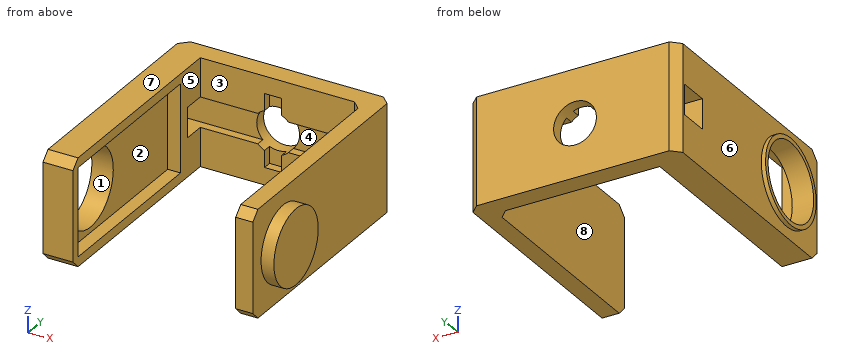
Autodesk Inventor part; units mm, degrees
ref_plane "YZ Plane" through (0, 0, 0) normal (1, 0, 0) x (0, 1, 0)
ref_plane "XZ Plane" through (0, 0, 0) normal (0, 1, 0) x (-1, 0, 0)
ref_plane "XY Plane" through (0, 0, 0) normal (0, 0, 1) x (1, 0, 0)
sketch "Boceto1" plane through (0, 0, 0) normal (0, 0, 1) x (1, 0, 0)
  line L0 (-12, 0) -> (-16, 0)
  line L1 (-16, 0) -> (-16, 55)
  line L2 (-16, 55) -> (-12, 55)
  line L3 (-12, 55) -> (-12, 0)
  line L4 (-12, 55) -> (-62, 55)
  line L5 (-62, 55) -> (-62, 50.3)
  line L6 (-62, 50.3) -> (-12, 50.3)
  line L7 (-12, 50.3) -> (-12, 55)
  line L8 (-62, 55) -> (-58, 55)
  line L9 (-58, 55) -> (-58, 0)
  line L10 (-58, 0) -> (-62, 0)
  line L11 (-62, 0) -> (-62, 55)
  dimension "d4" = 4
  dimension "d5" = 55
  dimension "d6" = 50
  dimension "d7" = 4.7
  dimension "d8" = 4
  dimension "d9" = 55
extrude "Extrusión1" add sketch "Boceto1" along normal blind 25
sketch "Boceto2" plane through (-58, 0, 0) normal (1, 0, 0) x (0, 0, -1)
  line L0 (-25, 0) -> (-25, 50.3)
  circle A0 centre (-12.5, 12) radius 9
  line L1 (0, 0) -> (-25, 0)
  dimension "d12" = 12.5
  dimension "d13" = 18
  dimension "d21" = 12
extrude "Extrusión2" cut sketch "Boceto2" against normal blind 15
sketch "Boceto3" plane through (-12, 0, 0) normal (1, 0, 0) x (0, 0, -1)
  line L0 (0, 0) -> (0, 55)
  line L1 (0, 0) -> (-25, 0)
  circle A0 centre (-12.5, 12) radius 8.75
  dimension "d16" = 17.5
  dimension "d17" = 12
  dimension "d18" = 12.5
extrude "Extrusión3" add sketch "Boceto3" along normal blind 3
sketch "Boceto4" plane through (-58, 0, 0) normal (1, 0, 0) x (0, 0, -1)
  circle A0 centre (-12.5, 12) radius 9
  line L0 (0, 50.3) -> (-25, 50.3)
  line L1 (-25, 0) -> (-25, 50.3)
  line L2 (0, 0) -> (-25, 0)
  line L3 (0, 0) -> (0, 50.3)
extrude "Extrusión4" add sketch "Boceto4" along normal blind 4
sketch "Boceto7" plane through (-62, 55, 0) normal (0, 1, 0) x (1, 0, 0)
  line L0 (50, 0) -> (0, 0)
  circle A0 centre (25, -12.5) radius 5
  line L1 (6.5, -9) -> (43.5, -9)
  line L2 (43.5, -9) -> (43.5, -16)
  line L3 (43.5, -16) -> (6.5, -16)
  line L4 (6.5, -16) -> (6.5, -9)
  line L5 (23, -4) -> (27, -4)
  line L6 (27, -4) -> (27, -21)
  line L7 (27, -21) -> (23, -21)
  line L8 (23, -21) -> (23, -4)
  line L9 (50, 0) -> (0, 0)
  point P0 (58, 0)
  point P1 (6.5, -12.5)
  point P2 (25, -9)
  point P3 (23, -12.5)
  point P4 (25, -4)
  point P5 (25, 0)
  dimension "d29" = 10
  dimension "d30" = 37
  dimension "d31" = 7
  dimension "d32" = 12.5
  dimension "d33" = 4
  dimension "d34" = 17
extrude "Extrusión6" cut sketch "Boceto7" against normal blind 10 contours A0 L3 L6 L1 | L1 L6 A0 | A0 L6 L3 | L6 L1 L8 A0 | L6 L3 L8 L1 | A0 L8 L3 L6 | L8 L1 A0 | L8 L3 A0 L1 | A0 L3 L8
sketch "Boceto8" plane through (-16, 50.3, 0) normal (0, -1, 0) x (1, 0, 0)
  line L0 (-39.5, 9) -> (-2.5, 9)
  line L1 (-39.5, 16) -> (-39.5, 9)
  line L2 (-2.5, 16) -> (-39.5, 16)
  line L3 (-2.5, 9) -> (-2.5, 16)
  circle A0 centre (-21, 12.5) radius 5
  line L4 (-23, 21) -> (-23, 4)
  line L5 (-23, 4) -> (-19, 4)
  line L6 (-19, 4) -> (-19, 21)
  line L7 (-19, 21) -> (-23, 21)
  point P0 (16, 0)
extrude "Extrusión8" cut sketch "Boceto8" against normal blind 2 contours L1 L2 A0 L0 | A0 L2 L4 L0 | L4 L2 L6 L0 | L6 L2 A0 L0 | A0 L2 L3 L0
sketch "Boceto9" plane through (-16, 50.3, 0) normal (0, -1, 0) x (1, 0, 0)
  line L0 (-19, 4) -> (-19, 21)
  line L1 (-23, 21) -> (-23, 4)
  line L2 (-23, 4) -> (-19, 4)
  line L3 (-19, 21) -> (-23, 21)
  point P0 (16, 0)
extrude "Extrusión9" cut sketch "Boceto9" against normal blind 2
sketch "Boceto10" plane through (-54, 0, 0) normal (1, 0, 0) x (0, 0, -1)
  line L0 (-16, 50.3) -> (-9, 50.3)
  line L1 (-9, 50.3) -> (-9, 48.8686)
  line L2 (-9, 48.8686) -> (-16, 48.8686)
  line L3 (-16, 48.8686) -> (-16, 50.3)
  dimension "d43" = 7
  dimension "d44" = 1.4314
extrude "Extrusión10" cut sketch "Boceto10" against normal blind 2
chamfer "Chaflán3" distance 2 angle 45 1 edges at (-16, 50.3, 12.5)
chamfer "Chaflán4" distance 2 angle 45 1 edges at (-12, 55, 12.5)
sketch "Boceto11" plane through (-16, 50.3, 0) normal (0, 1, 0) x (1, 0, 0)
  line L0 (2, -16) -> (2, -9)
  line L1 (-40, -16) -> (-43.5, -16)
  line L2 (4, -9) -> (4, -16)
  line L3 (-43.5, -9) -> (-40, -9)
  point P0 (16, 0)
sketch "Boceto14" plane through (-62, 0, 0) normal (-1, 0, 0) x (0, 0, 1)
  circle A0 centre (12.5, 12) radius 9
  line L0 (25, 55) -> (25, 0)
  line L1 (0, 55) -> (25, 55)
  line L2 (0, 55) -> (0, 0)
  line L3 (0, 0) -> (25, 0)
  circle A1 centre (12.5, 12) radius 10
extrude "Extrusión13" cut sketch "Boceto14" against normal blind 1 contours L0 L3 L2 L1
chamfer "Chaflán8" distance 2 angle 45 1 edges at (-61, 55, 12.5)
chamfer "Chaflán10" distance 2 angle 45 4 edges at (-57.5, 0, 0) (-57.5, 0, 25) (-14, 0, 25) (-14, 0, 0)
sketch "Boceto18" plane through (-54, 0, 0) normal (1, 0, 0) x (0, 0, -1)
  line L0 (-16, 50.3) -> (-9, 50.3)
  line L1 (-9, 50.3) -> (-9, 45.3)
  line L2 (-9, 45.3) -> (-16, 45.3)
  line L3 (-16, 45.3) -> (-16, 50.3)
  point P0 (0, 0)
extrude "Extrusión17" cut sketch "Boceto18" against normal blind 10
sketch "Boceto19" plane through (-55.5, 52.3, 16) normal (1, 0, 0) x (0, 0, -1)
  line L0 (0, -2) -> (7, -2)
  line L1 (7, -2) -> (7, 0)
  line L2 (7, 0) -> (0, 0)
  line L3 (0, -2) -> (0, 0)
  point P0 (16, -52.3)
extrude "Extrusión18" cut sketch "Boceto19" against normal blind 10
sketch "Boceto20" plane through (-54, 0, 0) normal (1, 0, 0) x (0, 0, -1)
  line L0 (-25, 50.3) -> (-16, 50.3)
  circle A0 centre (-12.5, 12) radius 9
  line L1 (-22.75, 42.5) -> (-2.25, 42.5)
  line L2 (-2.25, 42.5) -> (-2.25, 2)
  line L3 (-2.25, 2) -> (-22.75, 2)
  line L4 (-22.75, 2) -> (-22.75, 42.5)
  line L5 (-22.75, 42.5) -> (-2.25, 2) construction
  line L6 (-2.25, 42.5) -> (-22.75, 2) construction
  line L7 (-22.75, 42.5) -> (-2.25, 42.5) construction
  point P0 (0, 0)
  point P1 (-12.5, 22.25)
  point P2 (-12.5, 2)
  dimension "d100" = 20.5
  dimension "d102" = 40.5
  dimension "d103" = 10
extrude "Extrusión19" cut sketch "Boceto20" against normal blind 3
properties part number "Enlace2Base"
Build history of the part. All positions in model axes, mm. Face numbers are marked on the shaded views. A direction names the side the tool comes from. Round coordinates to 2 decimals unless told otherwise and drop trailing zeros. Loops run counter-clockwise (first coordinate to the right, second up) from the corner with the lowest first, then second, coordinate; pieces in that order, holes last. Notation, with made-up numbers: (26.5, 64) -> (44.5, 64) arc R26 cw to (44.5, 82) -> close; hole circle Ø4 at (48.5, -21). An arc over 180 degrees is marked (long way). Answer in a Markdown table with one row per item.
Item 1: Which spindle directions (+Z, -Z, +X, -X, +Y, -Y) get a long thin tool onto all of the face, cutting with end or side? Do the marked faces 1, 2, 3 and 4. Say none if no direction does.
Answers below:
| item | result |
|---|---|
| face 1 | -X |
| face 2 | none |
| face 3 | +Z, -Z, -Y |
| face 4 | -X, -Y |
Item 2: Drill centre lines: L1, parallel to X at y = 28, z = 18; L2, parallel to X at y = 21.5, z = 11.75; L3, parallel to Y at x = -60.35, z = 12.5. Where is each one in solid material? Low to high. Write a range as [from, to].
Answers below:
| item | result |
|---|---|
| L1 | x = [-61, -57], [-16, -12] |
| L2 | x = [-62, -57], [-16, -12] |
| L3 | y = [0, 3], [21, 45.3], [52.3, 53.65] |
Item 3: Saw through at C-C (x = -37). Write the cut outline in (y, z), and give its area (3 significant figures).
Answers below:
| item | result |
|---|---|
| outline | (50.3, 0) -> (55, 0) -> (55, 7.5) -> (52.3, 7.5) -> (52.3, 4) -> (50.3, 4) -> close; (50.3, 21) -> (52.3, 21) -> (52.3, 17.5) -> (55, 17.5) -> (55, 25) -> (50.3, 25) -> close |
| area | 56.5 mm² |
Item 4: Saw through at A-A (y = 37.5). Write the cut outline in (x, z).
Answers below:
| item | result |
|---|---|
| outline | (-61, 0) -> (-54, 0) -> (-54, 2.25) -> (-57, 2.25) -> (-57, 22.75) -> (-54, 22.75) -> (-54, 25) -> (-61, 25) -> close; (-16, 0) -> (-12, 0) -> (-12, 25) -> (-16, 25) -> close |
Item 5: Mould opens along X. For the marked faces 5, 6, 7 and 8 say: +X half, -X half, draft (parallel to the pull), parting line (faces both ways), or undercut.
Answers below:
| item | result |
|---|---|
| face 5 | undercut |
| face 6 | -X half |
| face 7 | draft |
| face 8 | undercut |
Item 6: Saw through at B-B (y = 12). Write the cut outline in (x, z).
Answers below:
| item | result |
|---|---|
| outline | (-62, 2.5) -> (-61, 2.5) -> (-61, 0) -> (-54, 0) -> (-54, 2.25) -> (-57, 2.25) -> (-57, 3.5) -> (-62, 3.5) -> close; (-62, 21.5) -> (-57, 21.5) -> (-57, 22.75) -> (-54, 22.75) -> (-54, 25) -> (-61, 25) -> (-61, 22.5) -> (-62, 22.5) -> close; (-16, 0) -> (-12, 0) -> (-12, 3.75) -> (-9, 3.75) -> (-9, 21.25) -> (-12, 21.25) -> (-12, 25) -> (-16, 25) -> close |
Item 7: Pin check, flat tips, straight feed: pin 1 (6 mm diameter, centred on x = -15.5, y = 36, fed in from -Z); pin 2 (1.6 mm diameter, centred on y = 51.5, z = 19.5, fed in from -X); pin 3 (8 mm diameter, centred on x = -37, z = 12.5, fed in from +Y); pin 4 (6 mm diameter, centred on y = 25.5, z = 15, fed in from +X). Stop position of each tip, or through.
Answers below:
| item | result |
|---|---|
| pin 1 | stops at z = 0 |
| pin 2 | stops at x = -61 |
| pin 3 | passes through |
| pin 4 | stops at x = -12 |
